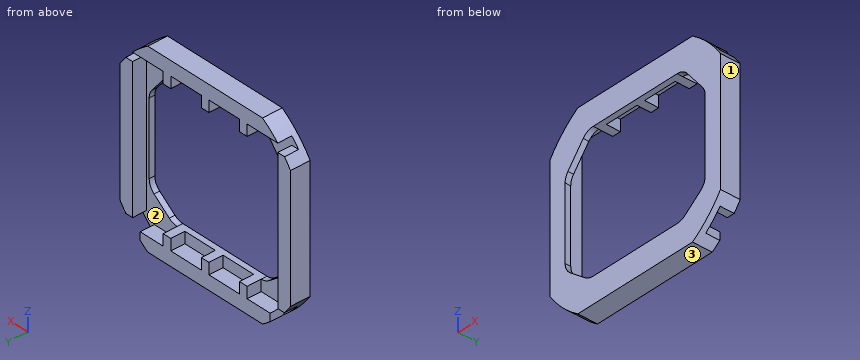
```python
from build123d import *

# Parameters (mm, degrees)
F0_W     = 67
F0_H     = 66
F1_DEPTH = 5
F2_W     = 67
F2_H     = 66
F3_DEPTH = 2
F4_W     = 12
F4_H     = 48
F5_DEPTH = 7.001
F7_DEPTH = 7.001
F8_W     = 6
F8_H     = 6
F9_DEPTH = 5


with BuildPart() as f1:
    # F0 (on Front) → F1 (new body)
    with BuildSketch(Plane.XZ):
        with Locations((28.5, 28)):
            Rectangle(F0_W, F0_H)
        Polygon((12, 0), (0, 0), (0, 56), (12, 56), (12, 52), (15, 52), (15, 56), (27, 56), (27, 52), (30, 52), (30, 56), (42, 56), (42, 52), (45, 52), (45, 56), (57, 56), (57, 0), (45, 0), (45, 4), (42, 4), (42, 0), (30, 0), (30, 4), (27, 4), (27, 0), (15, 0), (15, 4), (12, 4), align=None, mode=Mode.SUBTRACT)
    extrude(amount=F1_DEPTH)

    # F2 (on face) → F3 (join)
    with BuildSketch(Plane.XZ.offset(5)):
        with Locations((28.5, 28)):
            Rectangle(F2_W, F2_H)
        Polygon((12, 56), (12, 52), (15, 52), (15, 56), (27, 56), (27, 52), (30, 52), (30, 56), (42, 56), (42, 52), (45, 52), (45, 56), (57, 56), (57, 0), (45, 0), (45, 4), (42, 4), (42, 0), (30, 0), (30, 4), (27, 4), (27, 0), (15, 0), (15, 4), (12, 4), (12, 0), (0, 0), (0, 56), align=None, mode=Mode.SUBTRACT)
        Polygon((12, 4), (12, 52), (12, 56), (0, 56), (0, 0), (12, 0), align=None)
        Polygon((15, 56), (15, 52), (15, 4), (15, 0), (27, 0), (27, 4), (27, 52), (27, 56), align=None)
        Polygon((30, 56), (30, 52), (30, 4), (30, 0), (42, 0), (42, 4), (42, 52), (42, 56), align=None)
        Polygon((45, 56), (45, 52), (45, 4), (45, 0), (57, 0), (57, 56), align=None)
    extrude(amount=F3_DEPTH)

    # F4 (on face) → F5 (cut, through all)
    with BuildSketch(Plane.XZ.offset(7)):
        with BuildLine():
            Line((12, 4), (12, 52))
            ThreePointArc((12, 52), (9.834056, 51.506516), (8.095656, 50.123475))
            Line((8.095656, 50.123475), (2.095656, 42.623475))
            ThreePointArc((2.095656, 42.623475), (1.281858, 41.155035), (1, 39.5))
            Line((1, 39.5), (1, 13.691391))
            ThreePointArc((1, 13.691391), (1.505613, 11.50039), (2.920194, 9.752509))
            Line((2.920194, 9.752509), (8.920194, 5.061118))
            ThreePointArc((8.920194, 5.061118), (10.37126, 4.272717), (12, 4))
        make_face()
        with Locations((21, 28)):
            Rectangle(F4_W, F4_H)
        with Locations((36, 28)):
            Rectangle(F4_W, F4_H)
        with BuildLine():
            Line((56, 13.691391), (56, 39.5))
            ThreePointArc((56, 39.5), (55.718142, 41.155035), (54.904344, 42.623475))
            Line((54.904344, 42.623475), (48.904344, 50.123475))
            ThreePointArc((48.904344, 50.123475), (47.165944, 51.506516), (45, 52))
            Line((45, 52), (45, 4))
            ThreePointArc((45, 4), (46.62874, 4.272717), (48.079806, 5.061118))
            Line((48.079806, 5.061118), (54.079806, 9.752509))
            ThreePointArc((54.079806, 9.752509), (55.494387, 11.50039), (56, 13.691391))
        make_face()
    extrude(amount=-F5_DEPTH, mode=Mode.SUBTRACT)

    # F6 (on face) → F7 (cut, through all)
    with BuildSketch(Plane.XZ.offset(7)):
        with BuildLine():
            ThreePointArc((-5, 49.765856), (-0.066057, 55.928174), (5.983284, 61))
            Line((5.983284, 61), (-5, 61))
            Line((-5, 61), (-5, 49.765856))
        make_face()
        with BuildLine():
            Line((62, 61), (51.016716, 61))
            ThreePointArc((51.016716, 61), (57.066057, 55.928174), (62, 49.765856))
            Line((62, 49.765856), (62, 61))
        make_face()
        with BuildLine():
            Line((62, -5), (62, 6.234144))
            ThreePointArc((62, 6.234144), (57.066057, 0.071826), (51.016716, -5))
            Line((51.016716, -5), (62, -5))
        make_face()
        with BuildLine():
            ThreePointArc((5.983284, -5), (-0.066057, 0.071826), (-5, 6.234144))
            Line((-5, 6.234144), (-5, -5))
            Line((-5, -5), (5.983284, -5))
        make_face()
    extrude(amount=-F7_DEPTH, mode=Mode.SUBTRACT)

    # F8 (on face) → F9 (cut)
    with BuildSketch(Plane(origin=(0, 0, 0), x_dir=(-1, 0, 0), z_dir=(0, 1, 0))):
        with BuildLine():
            Line((-54, 59), (-60, 59))
            Line((-60, 59), (-60, 53))
            Line((-60, 53), (-54, 53))
            Line((-54, 53), (-54, 56))
            Line((-54, 56), (-56.995658, 56))
            ThreePointArc((-56.995658, 56), (-55.532899, 57.414705), (-54, 58.753089))
            Line((-54, 58.753089), (-54, 59))
        make_face()
        with BuildLine():
            Line((-3, 59), (-3, 58.753089))
            ThreePointArc((-3, 58.753089), (-1.467101, 57.414705), (-0.004342, 56))
            Line((-0.004342, 56), (-3, 56))
            Line((-3, 56), (-3, 53))
            Line((-3, 53), (3, 53))
            Line((3, 53), (3, 59))
            Line((3, 59), (-3, 59))
        make_face()
        Rectangle(F8_W, F8_H)
        with Locations((-57, 0)):
            Rectangle(F8_W, F8_H)
    extrude(amount=-F9_DEPTH, mode=Mode.SUBTRACT)


solid = f1.part
```
Input: part model. Units: mm. Frame: model coordinates. Face numbers are marked on the shaded views. Give positions to 0.01 mm unless a question says otherwise; leave off trailing zeros. Order: outer loops, then holes, each group sorted by start corner. A loop starts at its lowest first (then second) coordinate and runs counter-clockwise, first axis right, second up.
1. Mould query, pull axis X, two halves, no side actions, for the marked faces 1, 2 and 3. Classes: released by +X, released by -X, zero draft, split by the parting line, or undercut.
Derived:
face 1: released by +X
face 2: undercut
face 3: zero draft
2. Material intervals for L1, parallel to X at y = -3.75, z = 39; L2, parallel to Z at x = 10, y = -0.25; L3, parallel to Z at x = 42.5, y = -5.25, sorted ascending.
Derived:
L1: x = -5 to 0, 57 to 62
L2: z = -5 to 0, 56 to 61
L3: z = -5 to 4, 52 to 61
3. Section A-A on z = 36.5. Return the cut outline in (x, y), and give its area (3 significant figures).
Derived:
outline: (-5, -7) - (1, -7) - (1, -5) - (0, -5) - (0, 0) - (-5, 0) - close; (56, -7) - (62, -7) - (62, 0) - (57, 0) - (57, -5) - (56, -5) - close
area: 74.0 mm2
4. Section B-B on x = 43. Return the cut outline in (y, z).
Derived:
outline: (-7, -5) - (0, -5) - (0, 4) - (-7, 4) - close; (-7, 52) - (0, 52) - (0, 61) - (-7, 61) - close
5. Section D-D on x = 32. Return the cut outline in (y, z), and give its area (3 significant figures).
Derived:
outline: (-7, -5) - (0, -5) - (0, 0) - (-5, 0) - (-5, 4) - (-7, 4) - close; (-7, 52) - (-5, 52) - (-5, 56) - (0, 56) - (0, 61) - (-7, 61) - close
area: 86.0 mm2
6. Pin query (flat end, axial travel): pin 1 (1.2 mm diameter, centred on y = -2, z = 2, fed in from +X); pin 2 (1.4 mm diameter, centred on y = -3.5, z = -1, fed in from -X); pin 3 (0.8 mm diameter, centred on x = 58, y = -2, fed in from -Z). Return the tip coordinate at first contact, or that it passes through.
Derived:
pin 1: stops at x = 45
pin 2: stops at x = 3
pin 3: stops at z = 3
7. Section C-C on y = -6. Return the cut outline in (x, z), and give its area (3 significant figures).
Derived:
outline: (-5, 6.23) arc R39.95 ccw to (5.98, -5) - (51.02, -5) arc R39.95 ccw to (62, 6.23) - (62, 49.77) arc R39.95 ccw to (51.02, 61) - (5.98, 61) arc R39.95 ccw to (-5, 49.77) - close; hole (1, 13.69) arc R5 ccw to (2.92, 9.75) - (8.92, 5.06) arc R5 ccw to (12, 4) - (45, 4) arc R5 ccw to (48.08, 5.06) - (54.08, 9.75) arc R5 ccw to (56, 13.69) - (56, 39.5) arc R5 ccw to (54.9, 42.62) - (48.9, 50.12) arc R5 ccw to (45, 52) - (12, 52) arc R5 ccw to (8.1, 50.12) - (2.1, 42.62) arc R5 ccw to (1, 39.5) - close
area: 1,730 mm2
